Build history of the part. All positions in model axes, mm. A direction names the side the tool comes from. Coordinates: 2 decimals unless noted, no trailing zeros. Write each loop counter-clockwise with the first axis right and the second up, starting at its lowest first coordinate (ties: lowest second). Pieces come first, ordered by that corner, then holes.
```python
from build123d import *

# Parameters (mm, degrees)
F0_R     = 45.212
F1_DEPTH = 13.335
F2_R     = 2.5908
F3_DEPTH = 25.4
F4_R     = 14.5415
F5_DEPTH = 25.4
F7_DEPTH = 5.969
F8_R     = 28.829
F9_DEPTH = 4.826


with BuildPart() as f1:
    # F0 (on Top) → F1 (new body)
    with BuildSketch(Plane.XY):
        Circle(F0_R)
    extrude(amount=F1_DEPTH)

    # F2 (on face) → F3 (cut)
    with BuildSketch(Plane.XY.offset(13.335)):
        with Locations((-6.163129, 23.001109)):
            Circle(F2_R)
        with Locations((-23.001109, 6.163129)):
            Circle(F2_R)
        with Locations((-16.83798, -16.83798)):
            Circle(F2_R)
        with Locations((6.163129, -23.001109)):
            Circle(F2_R)
        with Locations((23.001109, -6.163129)):
            Circle(F2_R)
        with Locations((16.83798, 16.83798)):
            Circle(F2_R)
    extrude(amount=-F3_DEPTH, mode=Mode.SUBTRACT)

    # F4 (on face) → F5 (cut)
    with BuildSketch(Plane.XY.offset(13.335)):
        Circle(F4_R)
    extrude(amount=-F5_DEPTH, mode=Mode.SUBTRACT)

    # F6 (on face) → F7 (cut)
    with BuildSketch(Plane.XY.offset(13.335)):
        Polygon((-4.739815, 28.312987), (-10.051693, 26.889674), (-11.475007, 21.577795), (-7.586442, 17.68923), (-2.274564, 19.112544), (-0.85125, 24.424422), align=None)
        Polygon((22.149859, 18.261294), (18.261294, 22.149859), (12.949415, 20.726545), (11.526102, 15.414667), (15.414667, 11.526102), (20.726545, 12.949415), align=None)
        Polygon((26.889674, -10.051693), (28.312987, -4.739815), (24.424422, -0.85125), (19.112544, -2.274564), (17.68923, -7.586442), (21.577795, -11.475007), align=None)
        Polygon((4.739815, -28.312987), (10.051693, -26.889674), (11.475007, -21.577795), (7.586442, -17.68923), (2.274564, -19.112544), (0.85125, -24.424422), align=None)
        Polygon((-22.149859, -18.261294), (-18.261294, -22.149859), (-12.949415, -20.726545), (-11.526102, -15.414667), (-15.414667, -11.526102), (-20.726545, -12.949415), align=None)
        Polygon((-26.889674, 10.051693), (-28.312987, 4.739815), (-24.424422, 0.85125), (-19.112544, 2.274564), (-17.68923, 7.586442), (-21.577795, 11.475007), align=None)
    extrude(amount=-F7_DEPTH, mode=Mode.SUBTRACT)

    # F8 (on face) → F9 (cut)
    with BuildSketch(Plane(origin=(0, 0, 0), x_dir=(1, 0, 0), z_dir=(0, 0, -1))):
        Circle(F8_R)
    extrude(amount=-F9_DEPTH, mode=Mode.SUBTRACT)


solid = f1.part
```
1. Flat gauge pins, fed straight in: pin 1 (1 mm diameter, centred on y = 2.5, z = 4, fed in from -X); pin 2 (6.5 mm diameter, centred on x = 23, y = -6.16, fed in from +Z); pin 3 (4.5 mm diameter, centred on x = -16.84, y = -16.84, fed in from -Z); pin 4 (5.5 mm diameter, centred on x = -4, y = 21.5, fed in from +Z) (3 decimals). Where does each tip first touch, or does it go through?
Computed values:
pin 1: stops at x = -45.17
pin 2: stops at z = 7.37
pin 3: passes through
pin 4: stops at z = 13.335
2. 3-axis set-ups, long thin cutter, end or side, ignore diameter. For faces 3 (the face through (-6.25, 28.143, 2.379)), 4 (the face through (9.6, -19.7, 10.4)), 5 (the face through (19.31, 17.62, 6.11)): which of +Z, -Z, +X, -X, +Y, -Y reach the whole face in a straight line?
Computed values:
face 3: -Z
face 4: +Z
face 5: +Z, -Z
3. Saw through at C-C on x = -37. List the corners of the cut face in (y, z) (3 decimals).
Computed values:
outline: (-25.983, 0) - (25.983, 0) - (25.983, 13.335) - (-25.983, 13.335) - close
4. Saw through at D-D on y = -38. List the corners of the cut face in (x, z) (3 decimals), plus the area to 3 significant figures.
Computed values:
outline: (-24.497, 0) - (24.497, 0) - (24.497, 13.335) - (-24.497, 13.335) - close
area: 653 mm2
5. Saw through at B-B on z = 10.25. State how many separate pieces and enclosed holes the cut face has, plus the area to 3 significant figures.
Computed values:
separate pieces: 1
enclosed holes: 7
area: 5,290 mm2
6. Mould opens along X. For faces 1 (the face through (-1.573, 21.731, 10.392)), 2 (the face through (43.124, 13.58, 6.574)) say: +X half, -X half, draft (parallel to the pull), parting line (faces both ways), or undercut.
Computed values:
face 1: undercut
face 2: parting line
7. Probe line 1 along Y through (x, z) = (0, 10.25); line 2 along Z through (x, y) = (-9.5, 12) (3 decimals); line 3 along X through (y, z) = (-0.5, 3.75). List the from-to ranges inside material, lowest first.
Computed values:
line 1: y = -45.21 to -14.54, 14.54 to 45.21
line 2: z = 4.826 to 13.335
line 3: x = -45.21 to -28.82, 28.82 to 45.21
8. Saw through at A-A on z = 3.75. List the corners of the cut face in (x, y), plus the area to 3 significant figures.
Computed values:
outline: circle Ø90.42 at (0, 0); hole circle Ø57.66 at (0, 0)
area: 3,810 mm2
